For this review, take the finished solid that the model builds, in its own axes (mm). A direction names the side the tool comes from. Coordinates: 2 decimals unless noted, no trailing zeros. Write each loop counter-clockwise with the first axis right and the second up, starting at its lowest first coordinate (ties: lowest second). Pieces come first, ordered by that corner, then holes.
Autodesk Inventor part; units mm, degrees
ref_plane "YZ Plane" through (0, 0, 0) normal (1, 0, 0) x (0, 1, 0)
ref_plane "XZ Plane" through (0, 0, 0) normal (0, 1, 0) x (-1, 0, 0)
ref_plane "XY Plane" through (0, 0, 0) normal (0, 0, 1) x (1, 0, 0)
sketch "スケッチ1" plane through (0, 0, 0) normal (1, 0, 0) x (0, 1, 0)
  circle A0 centre (0, 0) radius 5
  circle A1 centre (0, 0) radius 15
  dimension "d0" = 10
  dimension "d1" = 30
extrude "押し出し1" add sketch "スケッチ1" along normal blind 9
sketch "スケッチ2" plane through (9, 0, 0) normal (1, 0, 0) x (0, 0, -1)
  circle A0 centre (0, 0) radius 14
  circle A1 centre (0, 0) radius 6
  dimension "d4" = 28
  dimension "d5" = 12
extrude "押し出し2" cut sketch "スケッチ2" against normal blind 0.1
sketch "スケッチ3" plane through (0, 0, 0) normal (-1, 0, 0) x (0, 0, 1)
  circle A0 centre (0, 0) radius 6
  circle A1 centre (0, 0) radius 14
  dimension "d8" = 12
  dimension "d9" = 28
extrude "押し出し3" cut sketch "スケッチ3" against normal blind 0.1
properties part number "Bearing_6200ZZ" material "鋼、炭素鋼"
1) Tool access review of faces 1 (the face through (0, -4, 4)), 2 (the face through (8.9, -6, -3)): name each direction out of +Z, -Z, +X, -X, +Y, -Y from which nothing blocks a thin tool from reaching the whole face with its end or side.
2) Consider section D-D (y = 11.5). Give the boundary of the cut face in (x, z), then the cut area to 3 significant figures.
3) Consider section A-A (y = 0). Give the boundary of the cut face in (x, z).
4) For L1, parallel to Y at x = 4.5, z = -0.25; L2, parallel to Z at x = 6.25, y = 0; L3, parallel to X at y = -8, z = 6.5, list the stretches that pass through material, from the lowest coordinate up.
5) The part is to be moulded in two halves that separate along Z. For faces 3 (the face through (0.1, -6, 3)), 4 (the face through (9, -4, 4)), 5 (the face through (4.44, -1.08, 4.88)), 6 (the face through (4.437, -14.985, -0.66)), say which applies: pulls with the +Z half, pulls with the -Z half, needs draft (parallel to the pull), parting line crosses it, or undercut.
6) Clearance check with flat-ended pins moving along their axes: P1, Ø1.5, axis at x = 6, y = -8, coming from the +Z side; P2, Ø5, axis at x = 2.5, y = -6.5, coming from the -Z side; P3, Ø1.5, axis at x = 7, z = 2.5, coming from the -Y side. State where each tip first meets the part, or that it passes through.
7) Consider section C-C (x = 1). Give the boundary of the cut face in (y, z), then the cut area to 3 significant figures.
Results:
1. face 1: +Z, -Z, -X, +Y, -Y
1. face 2: +X
2. outline: (0, -9.63) - (9, -9.63) - (9, -7.98) - (8.9, -7.98) - (8.9, 7.98) - (9, 7.98) - (9, 9.63) - (0, 9.63) - (0, 7.98) - (0.1, 7.98) - (0.1, -7.98) - (0, -7.98) - close
2. area: 170 mm2
3. outline: (0, -15) - (9, -15) - (9, -14) - (8.9, -14) - (8.9, -6) - (9, -6) - (9, -5) - (0, -5) - (0, -6) - (0.1, -6) - (0.1, -14) - (0, -14) - close; (0, 5) - (9, 5) - (9, 6) - (8.9, 6) - (8.9, 14) - (9, 14) - (9, 15) - (0, 15) - (0, 14) - (0.1, 14) - (0.1, 6) - (0, 6) - close
4. L1: y = -15 to -4.99, 4.99 to 15
4. L2: z = -15 to -5, 5 to 15
4. L3: x = 0.1 to 8.9
5. face 3: undercut
5. face 4: needs draft
5. face 5: undercut
5. face 6: parting line crosses it
6. P1: stops at z = 13.13
6. P2: stops at z = -14.46
6. P3: stops at y = -14.9
7. outline: circle Ø30 at (0, 0); hole circle Ø10 at (0, 0)
7. area: 628 mm2
